Geometry: final body of the model. Coordinates: model frame, mm. Give positions to 0.01 mm unless a question says otherwise; leave off trailing zeros. Loops run counter-clockwise (first coordinate to the right, second up) from the corner with the lowest first, then second, coordinate; pieces in that order, holes last. Notation, with made-up numbers: (9.5, 4) - (45.5, 4) arc R12 cw to (45.5, 26) - close; hole circle Ø4 at (-4, -31). An arc over 180 degrees is marked (long way). Use CSV: the item, a comma, the result in double quotes. Start each with the question number.
```python
from build123d import *

# Parameters (mm, degrees)
SKETCH1_W          = 400
SKETCH1_H          = 400
BASE_FLANGE1_DEPTH = 8
CUT_EXTRUDE1_DEPTH = 10


# Sheet-metal steps are written as plain solids
with BuildPart() as part:
    # Sketch1 → Base-Flange1 (new body)
    with BuildSketch(Plane(origin=(0, 0, 0), x_dir=(1, 0, 0), z_dir=(0, 1, 0))):
        with Locations((200, 200)):
            Rectangle(SKETCH1_W, SKETCH1_H)
    extrude(amount=-BASE_FLANGE1_DEPTH)

    # Sketch2 → Cut-Extrude1 (cut)
    with BuildSketch(Plane(origin=(0, 0, 0), x_dir=(1, 0, 0), z_dir=(0, 1, 0))):
        Polygon((80, 295), (80, 220), (20, 220), (20, 380), (80, 380), (80, 305), (92, 305), (92, 295), align=None)
        Polygon((92, 105), (80, 105), (80, 180), (20, 180), (20, 20), (80, 20), (80, 95), (92, 95), align=None)
        Polygon((320, 105), (320, 180), (380, 180), (380, 20), (320, 20), (320, 95), (308, 95), (308, 105), align=None)
        Polygon((308, 295), (320, 295), (320, 220), (380, 220), (380, 380), (320, 380), (320, 305), (308, 305), align=None)
    extrude(amount=-CUT_EXTRUDE1_DEPTH, mode=Mode.SUBTRACT)


solid = part.part
```
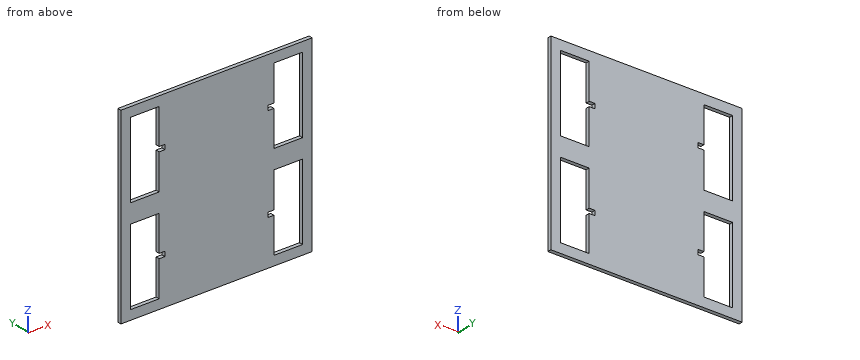
Item 1: Section B-B (z = -58.5). Output: boundary loops of the cut face in (x, y), plus the area to 3 significant figures.
Item 2: Section C-C (y = -1.5). Give the number of separate pieces and of enclosed holes in the cut face, plus the area to 3 significant figures.
Item 3: Ray query, probe 1 along X at (y, z) = (-3.75, -310.5); probe 2 along Z at (x, y) = (58.5, -4); probe 3 along Z at (x, y) = (86.5, -4.75). Return the intervals inside material, ascending.
Item 4: Section A-A (x = 339). Output: boundary loops of the cut face in (y, z).
Outcome:
1,outline,"(0, -8) - (20, -8) - (20, 0) - (0, 0) - close; (80, -8) - (320, -8) - (320, 0) - (80, 0) - close; (380, -8) - (400, -8) - (400, 0) - (380, 0) - close"
1,area,"2,240 mm2"
2,separate pieces,"1"
2,enclosed holes,"4"
2,area,"121,000 mm2"
3,probe 1,"x = 0 to 20, 80 to 320, 380 to 400"
3,probe 2,"z = -400 to -380, -220 to -180, -20 to 0"
3,probe 3,"z = -400 to -305, -295 to -105, -95 to 0"
4,outline,"(-8, -400) - (0, -400) - (0, -380) - (-8, -380) - close; (-8, -220) - (0, -220) - (0, -180) - (-8, -180) - close; (-8, -20) - (0, -20) - (0, 0) - (-8, 0) - close"
